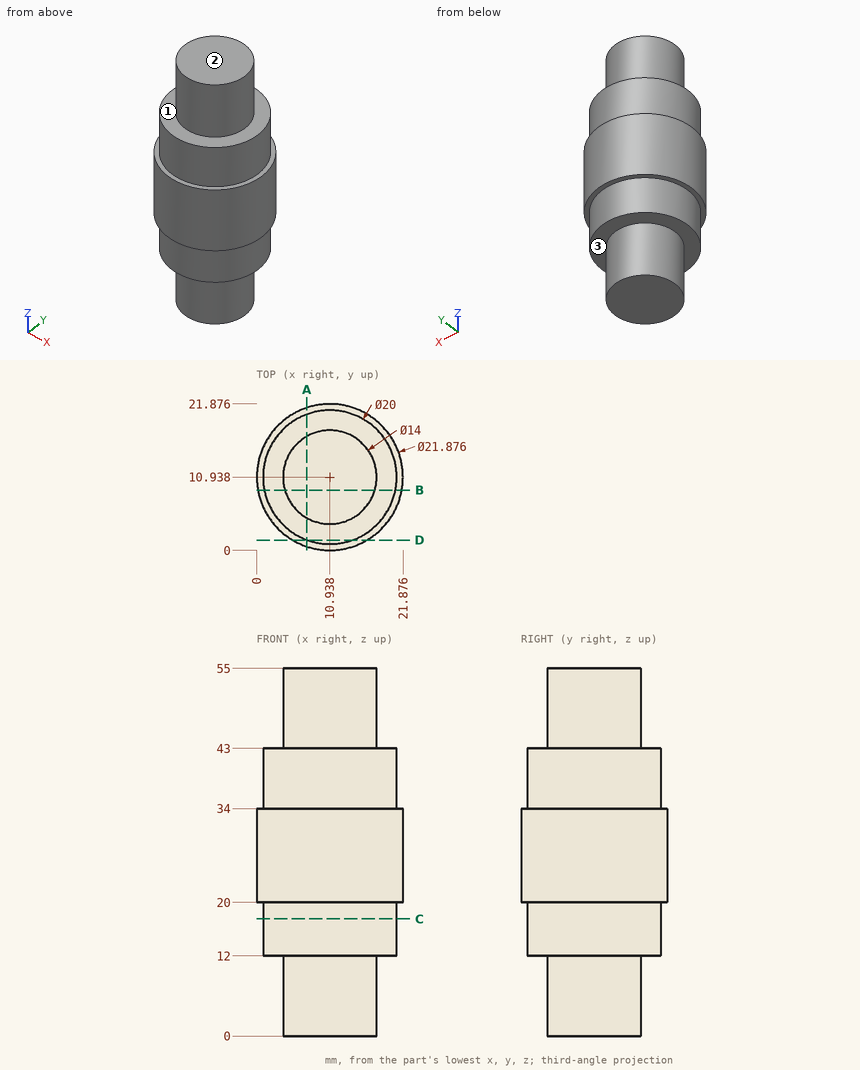
Here's the drawing with two shaded views (mm, measured from the low corner). I have some questions. A direction names the side the tool comes from. Give positions to 0.01 mm unless a question says otherwise; leave off trailing zeros. Order: outer loops, then holes, each group sorted by start corner. A loop starts at its lowest first (then second) coordinate and runs counter-clockwise, first axis right, second up. Notation, with made-up numbers: (1, 23.5) -> (43, 23.5) arc R23 cw to (43, 41.5) -> close; hole circle Ø3 at (88.25, -31.75). An arc over 180 degrees is marked (long way). Use a Markdown table: item, result. Add a question column.
Item 1: Imagine slicing it at C-C on z = 17.5. Please give me the cut outline in (x, y), plus the area to 3 significant figures.
Item 2: Imagine slicing it at B-B on y = 9. Please give me the cut outline in (x, z) (1 decimal), plus the area to 3 significant figures.
Item 3: For the marked faces 1, 2 and 3, which set-ups out of +Z, -Z, +X, -X, +Y, -Y let a thin tool reach every point of the face, with its end or its side?
Item 4: Will these pins go through, and if not, where does the flat tip stop? pin 1 (10 mm diameter, centred on x = 9.5, z = 11, fed in from -Y); pin 2 (12 mm diameter, centred on y = 10, z = 33, fed in from -X); pin 3 (8 mm diameter, centred on x = 17, z = 17, fed in from -Y); pin 4 (2 mm diameter, centred on x = 6.5, z = 25.5, fed in from +Y).
Item 5: Imagine slicing it at A-A on x = 7.5. Please give me the cut outline in (y, z) (1 decimal).
Item 6: I need wall thicknesses on line 1 (Z direction, x = 5.25, y = 17.75); line 2 (Y direction, x = 11.25, z = 43.5) (1 decimal); line 3 (Z direction, x = 17.25, y = 2.25). Which ranges of each line are inside material? Lowest first, please.
Item 7: Imagine slicing it at D-D on y = 1.5. Please give me the cut outline in (x, z), plus the area to 3 significant figures.
Data:
| question | item | result |
|---|---|---|
| 1 | outline | circle Ø20 at (10.94, 10.94) |
| 1 | area | 314 mm² |
| 2 | outline | (0.2, 20) -> (1.1, 20) -> (1.1, 12) -> (4.2, 12) -> (4.2, 0) -> (17.7, 0) -> (17.7, 12) -> (20.7, 12) -> (20.7, 20) -> (21.7, 20) -> (21.7, 34) -> (20.7, 34) -> (20.7, 43) -> (17.7, 43) -> (17.7, 55) -> (4.2, 55) -> (4.2, 43) -> (1.1, 43) -> (1.1, 34) -> (0.2, 34) -> close |
| 2 | area | 958 mm² |
| 3 | face 1 | +Z |
| 3 | face 2 | +Z, +X, -X, +Y, -Y |
| 3 | face 3 | -Z |
| 4 | pin 1 | stops at y = 0.94 |
| 4 | pin 2 | stops at x = 0 |
| 4 | pin 3 | stops at y = 0.55 |
| 4 | pin 4 | stops at y = 21.32 |
| 5 | outline | (0.6, 20) -> (1.5, 20) -> (1.5, 12) -> (4.8, 12) -> (4.8, 0) -> (17, 0) -> (17, 12) -> (20.3, 12) -> (20.3, 20) -> (21.3, 20) -> (21.3, 34) -> (20.3, 34) -> (20.3, 43) -> (17, 43) -> (17, 55) -> (4.8, 55) -> (4.8, 43) -> (1.5, 43) -> (1.5, 34) -> (0.6, 34) -> close |
| 6 | line 1 | z = 12 to 43 |
| 6 | line 2 | y = 3.9 to 17.9 |
| 6 | line 3 | z = 20 to 34 |
| 7 | outline | (5.41, 20) -> (7.63, 20) -> (7.63, 12) -> (14.24, 12) -> (14.24, 20) -> (16.47, 20) -> (16.47, 34) -> (14.24, 34) -> (14.24, 43) -> (7.63, 43) -> (7.63, 34) -> (5.41, 34) -> close |
| 7 | area | 267 mm² |
